Check sheet for the modelled part. Datum: model origin and axes. Units: mm. A direction names the side the tool comes from. Round coordinates to 2 decimals unless told otherwise and drop trailing zeros. Order: outer loops, then holes, each group sorted by start corner. A loop starts at its lowest first (then second) coordinate and runs counter-clockwise, first axis right, second up.
```python
from build123d import *

# Parameters (mm, degrees)
SKETCH2_W           = 1500
SKETCH2_H           = 1500
BOSS_EXTRUDE1_DEPTH = 10
SKETCH3_W           = 150
SKETCH3_H           = 20
SKETCH3_W_2         = 20
SKETCH3_H_2         = 1500
BOSS_EXTRUDE2_DEPTH = 110


with BuildPart() as part:
    # Sketch2 → Boss-Extrude1 (new body)
    with BuildSketch(Plane(origin=(0, 0, 0), x_dir=(1, 0, 0), z_dir=(0, 1, 0))):
        Rectangle(SKETCH2_W, SKETCH2_H)
    extrude(amount=BOSS_EXTRUDE1_DEPTH)

    # Sketch3 → Boss-Extrude2 (add)
    with BuildSketch(Plane(origin=(0, 10, 0), x_dir=(1, 0, 0), z_dir=(0, 1, 0))):
        Polygon((-600, 750), (-620, 750), (-620, -750), (-600, -750), (-600, -10), (-600, 10), align=None)
        with Locations((-525, 0)):
            Rectangle(SKETCH3_W, SKETCH3_H)
        with Locations((610, 0)):
            Rectangle(SKETCH3_W_2, SKETCH3_H_2)
    extrude(amount=BOSS_EXTRUDE2_DEPTH)


solid = part.part
```
Item 1: Sectioned sample at C-C (z = 556). Record the cut outline in (x, y), and give its area (3 significant figures).
Answer:
outline: (-750, 0) - (750, 0) - (750, 10) - (620, 10) - (620, 120) - (600, 120) - (600, 10) - (-600, 10) - (-600, 120) - (-620, 120) - (-620, 10) - (-750, 10) - close
area: 19,400 mm2
Item 2: Access from +Z, -Z, +X, -X, +Y, -Y to the whole of each face (thin tool, end or side, straight path). Record for faces 1 (the flat face through (-620, 64, -10)), 2 (the flat face through (684, 10, -10)), 3 (the flat face through (-600, 64, -375)), 4 (the flat face through (600, 64, 10)), 5 (the flat face through (-526, 64, 10)).
Answer:
face 1: +Z, -Z, -X, +Y
face 2: +Z, -Z, +X, +Y
face 3: -Z, +Y
face 4: +Z, -Z, +Y
face 5: +Z, +Y
Item 3: Sectioned sample at D-D (x = 270.5). Record the cut outline in (y, z), and give its area (3 significant figures).
Answer:
outline: (0, -750) - (10, -750) - (10, 750) - (0, 750) - close
area: 15,000 mm2
Item 4: Scan lines: line 1 along X through (y, z) = (86.5, -224); line 2 along Y through (x, z) = (-33, 123); line 3 along Z through (x, y) = (-532, 64.5). Record each from-to range of solid material in increasing order.
Answer:
line 1: x = -620 to -600, 600 to 620
line 2: y = 0 to 10
line 3: z = -10 to 10
Item 5: Sectioned sample at A-A (y = 40). Record the cut outline in (x, z), and give its area (3 significant figures).
Answer:
outline: (-620, -750) - (-600, -750) - (-600, -10) - (-450, -10) - (-450, 10) - (-600, 10) - (-600, 750) - (-620, 750) - close; (600, -750) - (620, -750) - (620, 750) - (600, 750) - close
area: 63,000 mm2
Item 6: Release check for a two-part mould opening along X. For faces 6 (the flat face through (-8, 10, -10)), 7 (the flat face through (-592, 120, -4)), 8 (the flat face through (620, 64, 10)) record: released by +X, released by -X, zero draft, split by the parting line, or undercut.
Answer:
face 6: undercut
face 7: zero draft
face 8: released by +X
Item 7: Go/stop test with flat-tipped pins: P1, Ø6, axis at x = 78.5, z = -359, coming from the +Y side; P2, Ø1, axis at y = 85.5, z = -196.5, coming from the -X side; P3, Ø22, axis at y = 82, z = -4.5, coming from the +X side. Record where each tip stops, or that it passes through.
Answer:
P1: stops at y = 10
P2: stops at x = -620
P3: stops at x = 620
Item 8: Sectioned sample at B-B (x = -491). Record the cut outline in (y, z).
Answer:
outline: (0, -750) - (10, -750) - (10, -10) - (120, -10) - (120, 10) - (10, 10) - (10, 750) - (0, 750) - close
